```python
from build123d import *

# Parameters (mm, degrees)
BOSS_EXTRU_1_DEPTH       = 21
ESQUISSE2_R              = 1
ENL_V_MAT_EXTRU_7_DEPTH  = 4
ESQUISSE6_R              = 1
ENL_V_MAT_EXTRU_8_DEPTH  = 4
ESQUISSE7_R              = 1
ENL_V_MAT_EXTRU_9_DEPTH  = 4
ESQUISSE8_R              = 1
ENL_V_MAT_EXTRU_10_DEPTH = 4


with BuildPart() as part:
    # Esquisse1 → Boss.-Extru.1 (new body)
    with BuildSketch(Plane.XY):
        with BuildLine():
            Line((-28.419332535, 4.995952024), (-10.419332535, 4.995952024))
            ThreePointArc((-10.419332535, 4.995952024), (-8.298012191, 4.117272368), (-7.419332535, 1.995952024))
            Line((-7.419332535, 1.995952024), (-7.419332535, -37.004047976))
            ThreePointArc((-7.419332535, -37.004047976), (-8.298012191, -39.12536832), (-10.419332535, -40.004047976))
            Line((-10.419332535, -40.004047976), (-28.419332535, -40.004047976))
            ThreePointArc((-28.419332535, -40.004047976), (-30.540652878, -39.12536832), (-31.419332535, -37.004047976))
            Line((-31.419332535, -37.004047976), (-31.419332535, 1.995952024))
            ThreePointArc((-31.419332535, 1.995952024), (-30.540652878, 4.117272368), (-28.419332535, 4.995952024))
        make_face()
    extrude(amount=BOSS_EXTRU_1_DEPTH)

    # Esquisse2 → Enlèv. mat.-Extru.7 (cut)
    with BuildSketch(Plane.XY.offset(21)):
        with Locations((-28.419332535, -37.004047976)):
            Circle(ESQUISSE2_R)
    extrude(amount=-ENL_V_MAT_EXTRU_7_DEPTH, mode=Mode.SUBTRACT)

    # Esquisse6 → Enlèv. mat.-Extru.8 (cut)
    with BuildSketch(Plane.XY.offset(21)):
        with Locations((-10.419332535, -37.004047976)):
            Circle(ESQUISSE6_R)
    extrude(amount=-ENL_V_MAT_EXTRU_8_DEPTH, mode=Mode.SUBTRACT)

    # Esquisse7 → Enlèv. mat.-Extru.9 (cut)
    with BuildSketch(Plane.XY.offset(21)):
        with Locations((-28.419332535, 1.995952024)):
            Circle(ESQUISSE7_R)
    extrude(amount=-ENL_V_MAT_EXTRU_9_DEPTH, mode=Mode.SUBTRACT)

    # Esquisse8 → Enlèv. mat.-Extru.10 (cut)
    with BuildSketch(Plane.XY.offset(21)):
        with Locations((-10.419332535, 1.995952024)):
            Circle(ESQUISSE8_R)
    extrude(amount=-ENL_V_MAT_EXTRU_10_DEPTH, mode=Mode.SUBTRACT)


solid = part.part
```
The model under review builds one solid part; all positions refer to its coordinate system, in mm. A direction names the side the tool comes from. Round coordinates to 2 decimals unless told otherwise and drop trailing zeros. One line per question, with ' | ' between items.
Item 1: For faces 1 (the face through (-29.16, -36.33, 19.03)), 2 (the face through (-31.419, -18, 10)), list the 3-axis set-ups (+Z, -Z, +X, -X, +Y, -Y) from which the entire face can be reached by the end or side of a thin tool; tool diameter is ignored.
Resolved:
face 1: +Z | face 2: +Z, -Z, -X, +Y, -Y
Item 2: To check wall thickness, follow probe 1 along X at (y, z) = (3.5, 8.5); probe 2 along Y at (x, z) = (-9.75, 3). State the ranges of each line that lie inside material, in increasing order.
Resolved:
probe 1: x = -31.02 to -7.82 | probe 2: y = -39.93 to 4.92
Item 3: The part is to be moulded in two halves that separate along X. For faces 3 (the face through (-7.419, -17, 10)), 4 (the face through (-30.517, -39.149, 10.353)), 5 (the face through (-10, 2, 17)), say which applies: pulls with the +X half, pulls with the -X half, needs draft (parallel to the pull), parting line crosses it, or undercut.
Resolved:
face 3: pulls with the +X half | face 4: pulls with the -X half | face 5: undercut
